```python
from build123d import *

# Parameters (mm, degrees)
SKETCH1_W           = 10
SKETCH1_H           = 10
BOSS_EXTRUDE2_DEPTH = 0.204346
SKETCH3_W           = 25
SKETCH3_H           = 25
BOSS_EXTRUDE3_DEPTH = 1.5875


with BuildPart() as part:
    # Sketch1 → Boss-Extrude2 (new body)
    with BuildSketch(Plane(origin=(0, 0, 0), x_dir=(1, 0, 0), z_dir=(0, 1, 0))):
        Polygon((3.5, 5), (0, 5), (0, 0), (3.5, 0), (3.5, 4.5), (5.25, 4.5), (5.25, 22.125), (4.75, 22.125), (4.75, 5), align=None)
        Polygon((3.503473693, 14), (0, 14), (0, 9), (3.503473693, 9), (3.503473693, 11.25), (4.378473693, 11.25), (4.378473693, 22.125), (3.878473693, 22.125), (3.878473693, 11.75), (3.503473693, 11.75), align=None)
        Polygon((3.503473693, 23), (0, 23), (0, 18), (3.503473693, 18), (3.503473693, 22.5), (5.576932067, 22.5), (5.576932067, 10.25), (17.5, 10.25), (17.5, 10.75), (6.125, 10.75), (6.125, 23), align=None)
        Polygon((18.5, 23.946155101), (18.5, 12), (6.5, 12), (6.5, 23.946155101), (0, 25), (25, 25), align=None)
        with Locations((12.5, 18)):
            Rectangle(SKETCH1_W, SKETCH1_H, mode=Mode.SUBTRACT)
        with Locations((12.5, 18)):
            Rectangle(SKETCH1_W, SKETCH1_H)
        Polygon((25, 18), (25, 23), (21.5, 23), (18.875, 23), (18.875, 11.625), (7.5, 11.625), (7.5, 11.125), (19.375, 11.125), (19.375, 22.5), (21.5, 22.5), (21.5, 18), align=None)
        Polygon((25, 9), (25, 14), (21.5, 14), (21.5, 11.75), (21.125, 11.75), (21.125, 22.125), (20.625, 22.125), (20.625, 11.25), (21.5, 11.25), (21.5, 9), align=None)
        Polygon((25, 0), (25, 5), (21.5, 5), (20.25, 5), (20.25, 22.125), (19.75, 22.125), (19.75, 4.5), (21.5, 4.5), (21.5, 0), align=None)
    extrude(amount=BOSS_EXTRUDE2_DEPTH)

    # Sketch3 → Boss-Extrude3 (add)
    with BuildSketch(Plane(origin=(0, 0, 0), x_dir=(1, 0, 0), z_dir=(0, 1, 0))):
        with Locations((12.5, 12.5)):
            Rectangle(SKETCH3_W, SKETCH3_H)
    extrude(amount=-BOSS_EXTRUDE3_DEPTH)


solid = part.part
```
Verification items for the finished model (mm, model axes). Give positions to 0.01 mm unless a question says otherwise; leave off trailing zeros. Loops run counter-clockwise (first coordinate to the right, second up) from the corner with the lowest first, then second, coordinate; pieces in that order, holes last. Notation, with made-up numbers: M -14,66 L 41,66 A28 ccw 41,101 Z; hole C -36.5,3 d5. An arc over 180 degrees is marked long. One line per question, with ' | ' between items.
Item 1: Draft check along Z on faces 1 (the face through (12, 0, -7)), 2 (the face through (23, 0.204, -13)), 3 (the face through (12, -1, -25)), 4 (the face through (12, -1, 0)). Enter one of: +Z half, -Z half, draft (parallel to the pull), parting line (faces both ways), or undercut.
Completed:
face 1: undercut | face 2: draft | face 3: -Z half | face 4: +Z half
Item 2: Thickness scan on line 1 (Z direction, x = 1.75, y = 0.05); line 2 (Z direction, x = 2.5, y = 0.15); line 3 (Y direction, x = 17.5, z = -2.5). Record the ranges inside material, lowest first. Write a range as [from, to].
Completed:
line 1: z = [-25, -24.72], [-23, -18], [-14, -9], [-5, 0] | line 2: z = [-25, -24.59], [-23, -18], [-14, -9], [-5, 0] | line 3: y = [-1.59, 0]
Item 3: Section check C-C, the plane x = 2.5. Record the cut outline in (y, z).
Completed:
outline: M -1.59,-25 L 0.2,-25 L 0.2,-24.59 L 0,-24.59 L 0,-23 L 0.2,-23 L 0.2,-18 L 0,-18 L 0,-14 L 0.2,-14 L 0.2,-9 L 0,-9 L 0,-5 L 0.2,-5 L 0.2,0 L -1.59,0 Z
